```python
from build123d import *

# Parameters (mm, degrees)
F1_DEPTH = 9
F0_W     = 5
F0_H     = 2
F2_DEPTH = 4.5
F3_R     = 2.1
F4_DEPTH = 11.001
F6_DEPTH = 11.001
F7_W     = 4.139266
F7_H     = 14
F7_W_2   = 3.360734
F8_DEPTH = 58
F9_R     = 1


with BuildPart() as f1:
    # F0 (on Top) → F1 (new body, symmetric)
    with BuildSketch(Plane.XY):
        Polygon((-49.633269, 10.227227), (-49.633269, 5.366493), (-32.633269, 5.366493), (-32.633269, 7.366493), (-21.633269, 7.366493), (-21.633269, 11.366493), (12.366731, 11.366493), (12.366731, 13.366493), (12.366731, 16.366493), (-29.633269, 16.366493), (-39.633269, 10.227227), align=None)
    extrude(amount=F1_DEPTH, both=True)

    # F0 (on Top) → F2 (join, symmetric)
    with BuildSketch(Plane.XY):
        with Locations((14.866731, 12.366493)):
            Rectangle(F0_W, F0_H)
    extrude(amount=F2_DEPTH, both=True)

    # F3 (on face) → F4 (cut, through all)
    with BuildSketch(Plane.XZ.offset(-5.366493)):
        with Locations((-41.133269, 0)):
            Circle(F3_R)
    extrude(amount=-F4_DEPTH, mode=Mode.SUBTRACT)

    # F5 (on face) → F6 (cut, through all)
    with BuildSketch(Plane(origin=(0, 16.366493, 0), x_dir=(-1, 0, 0), z_dir=(0, 1, 0))):
        with BuildLine():
            ThreePointArc((0.883269, 4.25), (-3.366731, 0), (0.883269, -4.25))
            Line((0.883269, -4.25), (29.534266, -4.25))
            Line((29.534266, -4.25), (29.633269, -4.25))
            Line((29.633269, -4.25), (29.633269, 4.25))
            Line((29.633269, 4.25), (29.534266, 4.25))
            Line((29.534266, 4.25), (0.883269, 4.25))
        make_face()
        Polygon((29.633269, 4.25), (29.633269, -4.25), (32.633269, -4.25), (32.642357, 4.25), align=None)
    extrude(amount=-F6_DEPTH, mode=Mode.SUBTRACT)

    # F7 (on face) → F8 (cut)
    with BuildSketch(Plane(origin=(-49.633269, 0, 0), x_dir=(0, -1, 0), z_dir=(-1, 0, 0))):
        with Locations((-12.29686, 0)):
            Rectangle(F7_W, F7_H)
        with Locations((-8.54686, 0)):
            Rectangle(F7_W_2, F7_H)
    extrude(amount=-F8_DEPTH, mode=Mode.SUBTRACT)

    # F9
    f9_edges = [f1.edges().sort_by_distance(p)[0] for p in [
        (-21.633269, 7.366493, 8),
        (-21.633269, 7.366493, -8),
    ]]
    fillet(f9_edges, radius=F9_R)


solid = f1.part
```
CAD build for the part. Positions are in the model's coordinates, mm. A direction names the side the tool comes from. Coordinates: 2 decimals unless noted, no trailing zeros. Order: outer loops, then holes, each group sorted by start corner. A loop starts at its lowest first (then second) coordinate and runs counter-clockwise, first axis right, second up.
(1) Which spindle directions (+Z, -Z, +X, -X, +Y, -Y) get a long thin tool onto all of the face, cutting with end or side? Do faces 5 (the face through (-19, 12, -9)), 6 (the face through (-32.633, 6, 7)), 7 (the face through (-45, 10.227, -8)). Say none if no direction does.
Solution:
face 5: -Z, +X, -X, +Y, -Y
face 6: +Z, -Z, +X, -Y
face 7: +Z, -Z, -X, +Y
(2) Mould opens along Z. For faces 1 (the face through (3.366, 15.38, 0.093)), 2 (the face through (15, 12, 4.5)), 3 (the face through (-17, 15, -4.25)), 4 (the face through (-45, 10.227, 8)) say: released by +Z, released by -Z, zero draft, split by the parting line, or undercut.
Solution:
face 1: undercut
face 2: released by +Z
face 3: undercut
face 4: zero draft
(3) Pin check, flat tips, straight feed: pin 1 Ø2.5 at (x, z) = (15.5, 1.5) entering from +Y; pin 2 Ø1.6 at (x, z) = (-43, -8) entering from +Y; pin 3 Ø1 at (y, z) = (6, 5.5) entering from +X; pin 4 Ø2 at (y, z) = (7, 6.5) entering from -X. Stop position of each tip, or through.
Solution:
pin 1: stops at y = 13.37
pin 2: stops at y = 10.23
pin 3: stops at x = -32.63
pin 4: stops at x = -49.63
(4) Drill centre lines: L1, parallel to Z at x = -19.5, y = 11.5; L2, parallel to Z at x = -2, y = 15.75; L3, parallel to Y at x = 9, z = -4.5. Where is each one in solid material? Low to high.
Solution:
L1: z = -9 to -7, 7 to 9
L2: z = -9 to -4.25, 4.25 to 9
L3: y = 11.37 to 16.37
(5) Saw through at C-C, the plane z = 0. Write the cut outline in (x, y).
Solution:
outline: (-49.63, 5.37) - (-43.23, 5.37) - (-43.23, 6.87) - (-49.63, 6.87) - close; (-39.03, 5.37) - (-32.64, 5.37) - (-32.64, 6.87) - (-39.03, 6.87) - close; (-32.89, 14.37) - (-32.64, 14.37) - (-32.64, 14.52) - close; (3.37, 14.37) - (8.37, 14.37) - (8.37, 11.37) - (17.37, 11.37) - (17.37, 13.37) - (12.37, 13.37) - (12.37, 16.37) - (3.37, 16.37) - close
(6) Saw through at A-A, the plane y = 9.5. Write the cut outline in (x, z), and give its area (3 significant figures).
Solution:
outline: (-49.63, -9) - (-21.63, -9) - (-21.63, -7) - (-49.63, -7) - close; (-49.63, 7) - (-21.63, 7) - (-21.63, 9) - (-49.63, 9) - close
area: 112 mm2
(7) Saw through at B-B, the plane x = -11. Write the cut outline in (y, z).
Solution:
outline: (11.37, -9) - (16.37, -9) - (16.37, -4.25) - (14.37, -4.25) - (14.37, -7) - (11.37, -7) - close; (11.37, 7) - (14.37, 7) - (14.37, 4.25) - (16.37, 4.25) - (16.37, 9) - (11.37, 9) - close
(8) Saw through at D-D, the plane x = -26.5. Write the cut outline in (y, z), and give its area (3 significant figures).
Solution:
outline: (7.37, -9) - (16.37, -9) - (16.37, -4.25) - (14.37, -4.25) - (14.37, -7) - (7.37, -7) - close; (7.37, 7) - (14.37, 7) - (14.37, 4.25) - (16.37, 4.25) - (16.37, 9) - (7.37, 9) - close
area: 47.0 mm2
